Could you check a few things on this model? Use its own coordinates, in mm. Give positions to 0.01 mm unless a question says otherwise; leave off trailing zeros. Order: outer loops, then holes, each group sorted by start corner. A loop starts at its lowest first (then second) coordinate and runs counter-clockwise, first axis right, second up. Notation, with made-up numbers: M 52.25,82 L 69.25,82 A22 cw 69.25,92 Z; hole C 2.5,88 d1. An arc over 180 degrees is marked long. Use a Markdown table: item, result. Add a question column.
Item 1: Suppose I cut it at A-A on z = -2.5. Write out the boundary of the cut face in (x, y), plus the area to 3 significant figures.
Item 2: I'm going to push flat-ended pins straight in: pin 1 Ø6 at (x, z) = (50.5, 2) entering from -Y; pin 2 Ø8 at (x, z) = (52, 6) entering from -Y; pin 3 Ø0.5 at (x, z) = (88, 9) entering from +Y. Where does each tip first touch, or does it pass through?
Item 3: Suppose I cut it at B-B on x = -66.5. Write out the boundary of the cut face in (y, z), plus the area to 3 significant figures.
Item 4: If I drill on L1, parallel to Z at x = -29, y = 0; L2, parallel to Y at x = 70, z = -0.75; L3, parallel to X at y = -41, z = 8.5, over which ranges is the centre line in solid material (lowest first)? Write a range as from..to.
from build123d import *

# Parameters (mm, degrees)
SKETCH3_R               = 11
SKETCH3_R_2             = 10.2
CUT_EXTRUDE1_REACH      = 196.756
SKETCH4_R               = 3.3
SKETCH5_R               = 3.3
CUT_EXTRUDE2_DEPTH      = 195.756456884
CUT_EXTRUDE3_DEPTH      = 195.756456884
CUT_EXTRUDE3_DEPTH_BACK = 195.756456884


with BuildPart() as part:
    # Sweep2: sweep along a path in Sketch1
    with BuildLine(Plane.XY) as sweep2_path:
        Line((132.955173363, 0), (88.955173363, 0))
        Line((88.955173363, 0), (-88.955173363, 0))
        ThreePointArc((-88.955173363, 0), (-120.695576987, -10.313082304), (-140.312225243, -37.313082304))
        Line((-140.312225243, -37.313082304), (-153.044826637, -76.5))
        Line((-153.044826637, -76.5), (-158.406001625, -93))
    # Sketch3 → Sweep2 (sweep)
    with BuildSketch(Plane(origin=(88.955173363, 0, 0), x_dir=(0, 0, -1), z_dir=(1, 0, 0))):
        Circle(SKETCH3_R)
        Circle(SKETCH3_R_2, mode=Mode.SUBTRACT)
    sweep(path=sweep2_path.line)

    # Sketch4 → Cut-Extrude1 (cut, up to next)
    with BuildSketch(Plane.XY, mode=Mode.PRIVATE) as cut_extrude1_sk1:
        with Locations(Location((-153.044826637, -76.5, 0), (0, 0, 162))):
            Circle(SKETCH4_R)
    cut_extrude1_tool1 = extrude(cut_extrude1_sk1.sketch, amount=CUT_EXTRUDE1_REACH, mode=Mode.PRIVATE) & part.part
    # Sketch4 → Cut-Extrude1 (cut, up to next)
    with BuildSketch(Plane.XY, mode=Mode.PRIVATE) as cut_extrude1_sk2:
        with BuildLine():
            Line((133.739588828, 2.555545653), (133.739588828, -2.555545653))
            Line((133.739588828, -2.555545653), (130.539588828, -2.555545653))
            ThreePointArc((130.539588828, -2.555545653), (129.125375266, -1.969759216), (128.539588828, -0.555545653))
            Line((128.539588828, -0.555545653), (128.539588828, 0.555545653))
            ThreePointArc((128.539588828, 0.555545653), (129.125375266, 1.969759216), (130.539588828, 2.555545653))
            Line((130.539588828, 2.555545653), (133.739588828, 2.555545653))
        make_face()
    cut_extrude1_tool2 = extrude(cut_extrude1_sk2.sketch, amount=CUT_EXTRUDE1_REACH, mode=Mode.PRIVATE) & part.part
    # Sketch4 → Cut-Extrude1 (cut, up to next)
    with BuildSketch(Plane.XY, mode=Mode.PRIVATE) as cut_extrude1_sk3:
        with BuildLine():
            Line((86.955173363, -5.5), (90.955173363, -5.5))
            ThreePointArc((90.955173363, -5.5), (92.369386925, -4.914213562), (92.955173363, -3.5))
            Line((92.955173363, -3.5), (92.955173363, 3.5))
            ThreePointArc((92.955173363, 3.5), (92.369386925, 4.914213562), (90.955173363, 5.5))
            Line((90.955173363, 5.5), (86.955173363, 5.5))
            ThreePointArc((86.955173363, 5.5), (85.540959801, 4.914213562), (84.955173363, 3.5))
            Line((84.955173363, 3.5), (84.955173363, -3.5))
            ThreePointArc((84.955173363, -3.5), (85.540959801, -4.914213562), (86.955173363, -5.5))
        make_face()
    cut_extrude1_tool3 = extrude(cut_extrude1_sk3.sketch, amount=CUT_EXTRUDE1_REACH, mode=Mode.PRIVATE) & part.part
    add(cut_extrude1_tool1.solids().sort_by_distance((-153.044827, -76.5, 0))[0], mode=Mode.SUBTRACT)
    add(cut_extrude1_tool2.solids().sort_by_distance((131.288287, 0, 0))[0], mode=Mode.SUBTRACT)
    add(cut_extrude1_tool3.solids().sort_by_distance((88.955173, 0, 0))[0], mode=Mode.SUBTRACT)

    # Sketch5 → Cut-Extrude2 (cut, through all)
    with BuildSketch(Plane.XY):
        with Locations(Location((-153.044826637, -76.5, 0), (0, 0, 162))):
            Circle(SKETCH5_R)
    extrude(amount=-CUT_EXTRUDE2_DEPTH, mode=Mode.SUBTRACT)

    # Sketch6 → Cut-Extrude3 (cut, two sides: drawn at the far end of the back side and taken through both)
    with BuildSketch(Plane.XY.offset(-CUT_EXTRUDE3_DEPTH_BACK)):
        with BuildLine():
            Line((132.955173363, 2.555545653), (129.755173363, 2.555545653))
            ThreePointArc((129.755173363, 2.555545653), (128.340959801, 1.969759216), (127.755173363, 0.555545653))
            Line((127.755173363, 0.555545653), (127.755173363, -0.555545653))
            ThreePointArc((127.755173363, -0.555545653), (128.340959801, -1.969759216), (129.755173363, -2.555545653))
            Line((129.755173363, -2.555545653), (132.955173363, -2.555545653))
            Line((132.955173363, -2.555545653), (132.955173363, 2.555545653))
        make_face()
    extrude(amount=CUT_EXTRUDE3_DEPTH + CUT_EXTRUDE3_DEPTH_BACK, mode=Mode.SUBTRACT)


solid = part.part
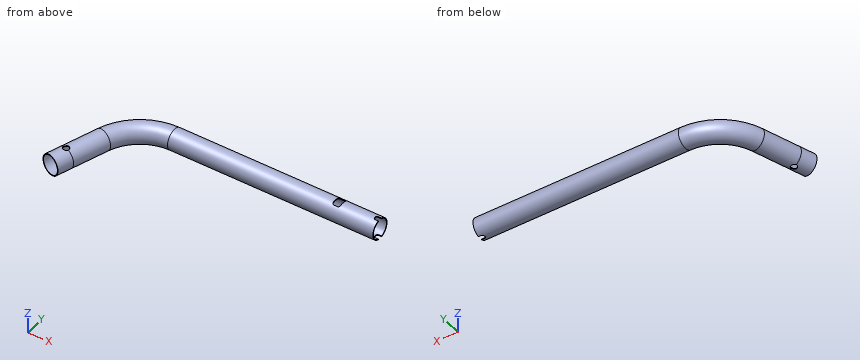
Findings below:
| question | item | result |
|---|---|---|
| 1 | outline | M -168.59,-89.69 L -167.81,-89.94 L -149.72,-34.26 A63.89 cw -88.96,9.89 L 132.96,9.89 L 132.96,10.71 L -88.96,10.71 A64.71 ccw -150.5,-34 Z; M -149,-96.06 L -148.22,-96.31 L -130.12,-40.62 A43.29 cw -88.96,-10.71 L 132.96,-10.71 L 132.96,-9.89 L -88.96,-9.89 A44.11 ccw -130.91,-40.37 Z |
| 1 | area | 574 mm^2 |
| 2 | pin 1 | stops at y = -11 |
| 2 | pin 2 | stops at y = -10.82 |
| 2 | pin 3 | stops at y = 6.67 |
| 3 | outline | C 0,0 d22; hole C 0,0 d20.4 |
| 3 | area | 53.3 mm^2 |
| 4 | L1 | z = -11..-10.2, 10.2..11 |
| 4 | L2 | y = -10.97..-10.17, 10.17..10.97 |
| 4 | L3 | x = -148.85..-147.44, -135.58..-134.17 |
